```python
from build123d import *

# Parameters (mm, degrees)
BOSS_EXTRUDE1_DEPTH = 27
SKETCH2_W           = 32
SKETCH2_H           = 22
CUT_EXTRUDE1_DEPTH  = 209.158593385


with BuildPart() as part:
    # Sketch1 → Boss-Extrude1 (new, symmetric)
    with BuildSketch(Plane.XY):
        with BuildLine():
            Line((0, 0), (10, 0))
            ThreePointArc((10, 0), (12.121320344, 0.878679656), (13, 3))
            Line((13, 3), (13, 6.867571163))
            Line((13, 6.867571163), (94, 6.867571163))
            Line((94, 6.867571163), (94, 3))
            ThreePointArc((94, 3), (94.878679656, 0.878679656), (97, 0))
            Line((97, 0), (103, 0))
            ThreePointArc((103, 0), (105.121320344, 0.878679656), (106, 3))
            Line((106, 3), (106, 6.867571163))
            Line((106, 6.867571163), (187, 6.867571163))
            Line((187, 6.867571163), (187, 3))
            ThreePointArc((187, 3), (187.878679656, 0.878679656), (190, 0))
            Line((190, 0), (200, 0))
            Line((200, 0), (200, 25))
            Line((200, 25), (145, 25))
            ThreePointArc((145, 25), (135.807611845, 28.807611845), (132, 38))
            Line((132, 38), (132, 76))
            Line((132, 76), (119, 76))
            Line((119, 76), (119, 44))
            ThreePointArc((119, 44), (100, 25), (81, 44))
            Line((81, 44), (81, 76))
            Line((81, 76), (68, 76))
            Line((68, 76), (68, 38))
            ThreePointArc((68, 38), (64.192388155, 28.807611845), (55, 25))
            Line((55, 25), (0, 25))
            Line((0, 25), (0, 0))
        make_face()
    extrude(amount=BOSS_EXTRUDE1_DEPTH, both=True)

    # Sketch2 → Cut-Extrude1 (cut, through all)
    with BuildSketch(Plane(origin=(0, 25, 0), x_dir=(1, 0, 0), z_dir=(0, 1, 0))):
        with Locations((34.218039328, 0)):
            Rectangle(SKETCH2_W, SKETCH2_H)
    cut_extrude1 = extrude(amount=-CUT_EXTRUDE1_DEPTH, mode=Mode.SUBTRACT)

    # Mirror1: Cut-Extrude1 across plane
    add(cut_extrude1.mirror(Plane(origin=(100, 0, 0), x_dir=(0, 0, 1), z_dir=(1, 0, 0))), mode=Mode.SUBTRACT)


solid = part.part
```
Geometry check sheet. Reference: the model listing, model coordinates, mm. A direction names the side the tool comes from. Round coordinates to 2 decimals unless told otherwise and drop trailing zeros. Order: outer loops, then holes, each group sorted by start corner. A loop starts at its lowest first (then second) coordinate and runs counter-clockwise, first axis right, second up. Notation, with made-up numbers: (29.25, 11) - (70.25, 11) arc R27 ccw to (70.25, 27) - close; hole circle Ø2 at (-32.5, 66). An arc over 180 degrees is marked (long way). Use a Markdown table: item, result. Add a question column.
(1) Sectioned sample at A-A, the plane y = 50. Enter the section's corners in (x, z).
(2) Tool access check on faces 4 (the flat face through (185, 25, 0)), 5 (the flat face through (146, 6.868, 0)), 6 (the flat face through (149.782, 16, 0)). Record the directions out of +Z, -Z, +X, -X, +Y, -Y that give a thin tool (end or side, any length) a straight path to the whole face; none if there is none.
(3) Depth check by flat-ended pin: pin 1 (5 mm diameter, centred on y = 38, z = 20.5, fed in from +X); pin 2 (16 mm diameter, centred on y = 59.5, z = 13, fed in from +X); pin 3 (1 mm diameter, centred on x = 99, z = -8, fed in from +Y); pin 4 (9 mm diameter, centred on y = 16, z = 5.5, fed in from -X). Enter the tip coordinate at first touch or a pass-through.
(4) Sectioned sample at C-C, the plane z = 6.5. Count the separate pieces of the cut face and the enclosed holes in it, and give its area (3 significant figures).
(5) Release check for a two-part mould opening along Z. For faces 1 (the flat face through (0, 13, 0)), 2 (the flat face through (34, 16, -11)), 3 (the flat face through (99, 22, 27)) record: pulls with the +Z half, pulls with the -Z half, needs draft (parallel to the pull), parting line crosses it, or undercut.
(6) Sectioned sample at D-D, the plane z = 15.5. Enter the section's corners in (x, y).
(7) Sectioned sample at B-B, the plane y = 9. Enter the section's corners in (x, z).
(8) Material ranges on line 1 along X through (y, z) = (5.5, 22); line 2 along X through (y, z) = (14, -3); line 3 along X through (y, z) = (52, 4), recorded low to high. Write a range as [from, to].
Answers below:
| question | item | result |
|---|---|---|
| 1 | outline | (68, -27) - (81, -27) - (81, 27) - (68, 27) - close; (119, -27) - (132, -27) - (132, 27) - (119, 27) - close |
| 2 | face 4 | +Z, -Z, +X, +Y |
| 2 | face 5 | +Z, -Z, -Y |
| 2 | face 6 | +Y, -Y |
| 3 | pin 1 | x = 132.24 |
| 3 | pin 2 | x = 132 |
| 3 | pin 3 | y = 25.06 |
| 3 | pin 4 | x = 0 |
| 4 | separate pieces | 3 |
| 4 | enclosed holes | 0 |
| 4 | area | 4,270 mm² |
| 5 | face 1 | needs draft |
| 5 | face 2 | undercut |
| 5 | face 3 | pulls with the +Z half |
| 6 | outline | (0, 0) - (10, 0) arc R3 ccw to (13, 3) - (13, 6.87) - (94, 6.87) - (94, 3) arc R3 ccw to (97, 0) - (103, 0) arc R3 ccw to (106, 3) - (106, 6.87) - (187, 6.87) - (187, 3) arc R3 ccw to (190, 0) - (200, 0) - (200, 25) - (145, 25) arc R13 cw to (132, 38) - (132, 76) - (119, 76) - (119, 44) arc R19 cw to (81, 44) - (81, 76) - (68, 76) - (68, 38) arc R13 cw to (55, 25) - (0, 25) - close |
| 7 | outline | (0, -27) - (200, -27) - (200, 27) - (0, 27) - close; hole (18.22, -11) - (50.22, -11) - (50.22, 11) - (18.22, 11) - close; hole (149.78, -11) - (181.78, -11) - (181.78, 11) - (149.78, 11) - close |
| 8 | line 1 | [0, 13], [94, 106], [187, 200] |
| 8 | line 2 | [0, 18.22], [50.22, 149.78], [181.78, 200] |
| 8 | line 3 | [68, 81], [119, 132] |
